Input: part model. Units: mm. Frame: model coordinates. Face numbers are marked on the shaded views. A direction names the side the tool comes from. Round coordinates to 2 decimals unless told otherwise and drop trailing zeros. Loops run counter-clockwise (first coordinate to the right, second up) from the corner with the lowest first, then second, coordinate; pieces in that order, holes last. Notation, with made-up numbers: M 8,-25.5 L 56,-25.5 A9 ccw 56,-8.5 Z; hole C 32.5,19.25 d8. An arc over 180 degrees is marked long. Return JSON: item names as keys, results as strings. Group by question number.
1) Section B-B (y = 3). Count the separate pieces of the cut face and the enclosed holes in it, plus the area to 3 significant figures.
2) Access query for the marked faces 4 and 5. Directions: +Z, -Z, +X, -X, +Y, -Y. A direction counts if a zero-diameter tool reaches every point of the face in a straight line with its end or side. Return the directions, or none.
3) Material intervals for line 1 (Z direction, x = 7.5, y = 3.85); line 2 (X direction, y = 2, z = -8.5); line 3 (Z direction, x = 4.5, y = 2.25), sorted ascending. Write a range as from..to.
4) Section A-A (x = 23). Output: boundary loops of the cut face in (y, z).
5) Section D-D (x = 4.5). Output: boundary loops of the cut face in (y, z), plus the area to 3 significant figures.
6) Contact query for flat-ended pins moving along their axis: P1, Ø2, axis at x = 12, z = 14, coming from the -Y side; P2, Ø1.1, axis at x = 24.5, z = 21.5, coming from the -Y side; P3, Ø1, axis at x = -8.5, z = -10.5, coming from the -Y side; P4, Ø1.3, axis at x = -4.78, z = -10.82, coming from the -Y side. Output: stop coordinate, or through.
7) Section C-C (z = 8.5). Output: boundary loops of the cut face in (x, y), plus the area to 3 significant figures.
8) Mould query, pull axis X, two halves, no side actions, for the marked faces 1, 2 and 3. Classes: +X half, -X half, draft (parallel to the pull), parting line (faces both ways), or undercut.
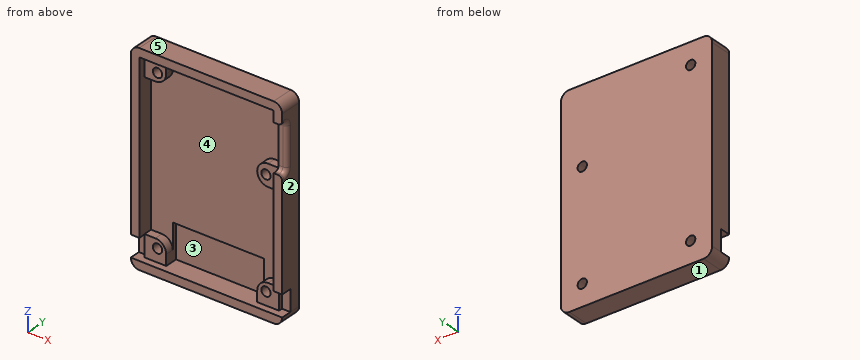
from build123d import *

# Parameters (mm, degrees)
SKETCH1_W           = 35.5
SKETCH1_H           = 48.2
SKETCH1_R           = 1.09
BOSS_EXTRUDE2_DEPTH = 5.2
SKETCH1_4_W         = 31.5
SKETCH1_4_H         = 44.2
CUT_EXTRUDE1_DEPTH  = 1.6
CUT_EXTRUDE2_DEPTH  = 2
SKETCH6_W           = 21.34
SKETCH6_H           = 8.5
CUT_EXTRUDE5_DEPTH  = 1
SKETCH4_W           = 2
SKETCH4_H           = 5
CUT_EXTRUDE3_DEPTH  = 2.5
SKETCH5_W           = 11
SKETCH5_H           = 1.5
CUT_EXTRUDE4_DEPTH  = 2
FILLET1_R           = 2
FILLET3_R           = 2.54
FILLET4_R           = 1
FILLET2_R           = 1


with BuildPart() as part:
    # Sketch1 → Boss-Extrude2 (new body)
    with BuildSketch(Plane(origin=(0, 0, 0), x_dir=(1, 0, 0), z_dir=(0, 1, 0))):
        with Locations((7.932292683, -8.236727254)):
            Rectangle(SKETCH1_W, SKETCH1_H)
        with Locations(Location((20.642292683, 10.823272746, 0), (0, 0, 270))):
            Circle(SKETCH1_R, mode=Mode.SUBTRACT)
        with Locations(Location((-4.777707317, 10.823272746, 0), (0, 0, 270))):
            Circle(SKETCH1_R, mode=Mode.SUBTRACT)
        with Locations(Location((-4.777707317, -27.296727254, 0), (0, 0, 270))):
            Circle(SKETCH1_R, mode=Mode.SUBTRACT)
        with Locations(Location((20.642292683, -14.576727254, 0), (0, 0, 270))):
            Circle(SKETCH1_R, mode=Mode.SUBTRACT)
    extrude(amount=BOSS_EXTRUDE2_DEPTH)

    # Sketch1<4> → Cut-Extrude1 (cut)
    with BuildSketch(Plane(origin=(0, 0, 0), x_dir=(1, 0, 0), z_dir=(0, 1, 0))):
        with Locations((7.932292683, -8.236727254)):
            Rectangle(SKETCH1_4_W, SKETCH1_4_H)
    extrude(amount=CUT_EXTRUDE1_DEPTH, mode=Mode.SUBTRACT)

    # Sketch3 → Cut-Extrude2 (cut)
    with BuildSketch(Plane.XZ.offset(-1.6)):
        Polygon((-2.737707317, -13.863272746), (18.602292683, -13.863272746), (18.602292683, -8.783272746), (23.682292683, -8.783272746), (23.682292683, 12.036727254), (18.602292683, 12.036727254), (18.602292683, 17.116727254), (23.682292683, 17.116727254), (23.682292683, 30.336727254), (-2.737707317, 30.336727254), (-2.737707317, 25.256727254), (-7.817707317, 25.256727254), (-7.817707317, -8.783272746), (-2.737707317, -8.783272746), align=None)
    extrude(amount=-CUT_EXTRUDE2_DEPTH, mode=Mode.SUBTRACT)

    # Sketch6 → Cut-Extrude5 (cut)
    with BuildSketch(Plane.XZ.offset(-3.6)):
        with Locations((7.932292683, -9.613272746)):
            Rectangle(SKETCH6_W, SKETCH6_H)
    extrude(amount=-CUT_EXTRUDE5_DEPTH, mode=Mode.SUBTRACT)

    # Sketch4 → Cut-Extrude3 (cut)
    with BuildSketch(Plane.XZ):
        with Locations((24.682292683, -11.363272746)):
            Rectangle(SKETCH4_W, SKETCH4_H)
        with Locations((-8.817707317, -11.363272746)):
            Rectangle(SKETCH4_W, SKETCH4_H)
    extrude(amount=-CUT_EXTRUDE3_DEPTH, mode=Mode.SUBTRACT)

    # Sketch5 → Cut-Extrude4 (cut)
    with BuildSketch(Plane(origin=(25.682292683, 0, 0), x_dir=(0, 0, -1), z_dir=(1, 0, 0))):
        with Locations((-22.236727254, 0.75)):
            Rectangle(SKETCH5_W, SKETCH5_H)
    extrude(amount=-CUT_EXTRUDE4_DEPTH, mode=Mode.SUBTRACT)

    # Fillet1
    fillet1_edges = [part.edges().sort_by_distance(p)[0] for p in [
        (-9.817707317, 2.6, -15.863272746),
        (25.682292683, 2.6, -15.863272746),
        (25.682292683, 2.6, 32.336727254),
        (-9.817707317, 2.6, 32.336727254),
    ]]
    fillet(fillet1_edges, radius=FILLET1_R - 0.0001)  # a hair under: the kernel refuses the full size

    # Fillet3
    fillet3_edges = [part.edges().sort_by_distance(p)[0] for p in [
        (-2.737707317, 2.6, 25.256727254),
        (18.602292683, 2.6, 17.116727254),
        (18.602292683, 2.6, 12.036727254),
        (18.602292683, 2.6, -8.783272746),
        (-2.737707317, 2.6, -8.783272746),
    ]]
    fillet(fillet3_edges, radius=FILLET3_R - 0.0001)  # a hair under: the kernel refuses the full size

    # Fillet4
    fillet4_edges = [part.edges().sort_by_distance(p)[0] for p in [
        (24.682292683, 1.5, 27.736727254),
        (24.682292683, 1.5, 16.736727254),
    ]]
    fillet(fillet4_edges, radius=FILLET4_R)

    # Fillet2
    fillet2_edges = [part.edges().sort_by_distance(p)[0] for p in [
        (25.682292683, 0.25, 16.736727254),
        (25.682292683, 0.25, 27.736727254),
        (25.682292683, 1.5, 22.236727254),
        (25.682292683, 1.207106781, 27.443834036),
        (25.682292683, 1.207106781, 17.029620473),
    ]]
    fillet(fillet2_edges, radius=FILLET2_R)


solid = part.part
Returned:
{
 "1": {"separate pieces": "1", "enclosed holes": "5", "area": "397 mm^2"},
 "2": {"face 4": "-Y", "face 5": "+Z, +X, -X, +Y, -Y"},
 "3": {"line 1": "z = -15.86..-13.86, -5.36..32.34", "line 2": "x = -9.82..-7.82, 23.68..25.68", "line 3": "z = -15.86..-13.86, 30.34..32.34"},
 "4": {"outline": "M 0,-15.86 L 5.2,-15.86 L 5.2,32.34 L 0,32.34 L 0,30.34 L 3.6,30.34 L 3.6,17.12 L 1.6,17.12 L 1.6,12.04 L 3.6,12.04 L 3.6,-8.78 L 1.6,-8.78 L 1.6,-13.86 L 0,-13.86 Z"},
 "5": {"outline": "M 0,-15.86 L 5.2,-15.86 L 5.2,32.34 L 0,32.34 L 0,30.34 L 3.6,30.34 L 3.6,-5.36 L 4.6,-5.36 L 4.6,-13.86 L 0,-13.86 Z", "area": "83.0 mm^2"},
 "6": {"P1": "stops at y = 3.6", "P2": "stops at y = 1.5", "P3": "stops at y = 2.5", "P4": "passes through"},
 "7": {"outline": "M -9.82,0 L -7.82,0 L -7.82,3.6 L 23.68,3.6 L 23.68,0 L 25.68,0 L 25.68,5.2 L -9.82,5.2 Z", "area": "71.2 mm^2"},
 "8": {"face 1": "draft", "face 2": "+X half", "face 3": "undercut"}
}
